The drawing under review shows one solid part. Ordinate dimensions are in mm from its lowest x, y, z. Coordinates: 2 decimals unless noted, no trailing zeros. Order: outer loops, then holes, each group sorted by start corner. A loop starts at its lowest first (then second) coordinate and runs counter-clockwise, first axis right, second up. Notation, with made-up numbers: (19.5, 49) - (36.5, 49) arc R25 ccw to (36.5, 82) - close; hole circle Ø11 at (66, 71.25). An arc over 180 degrees is marked (long way). Answer in a Markdown table with one row per item.
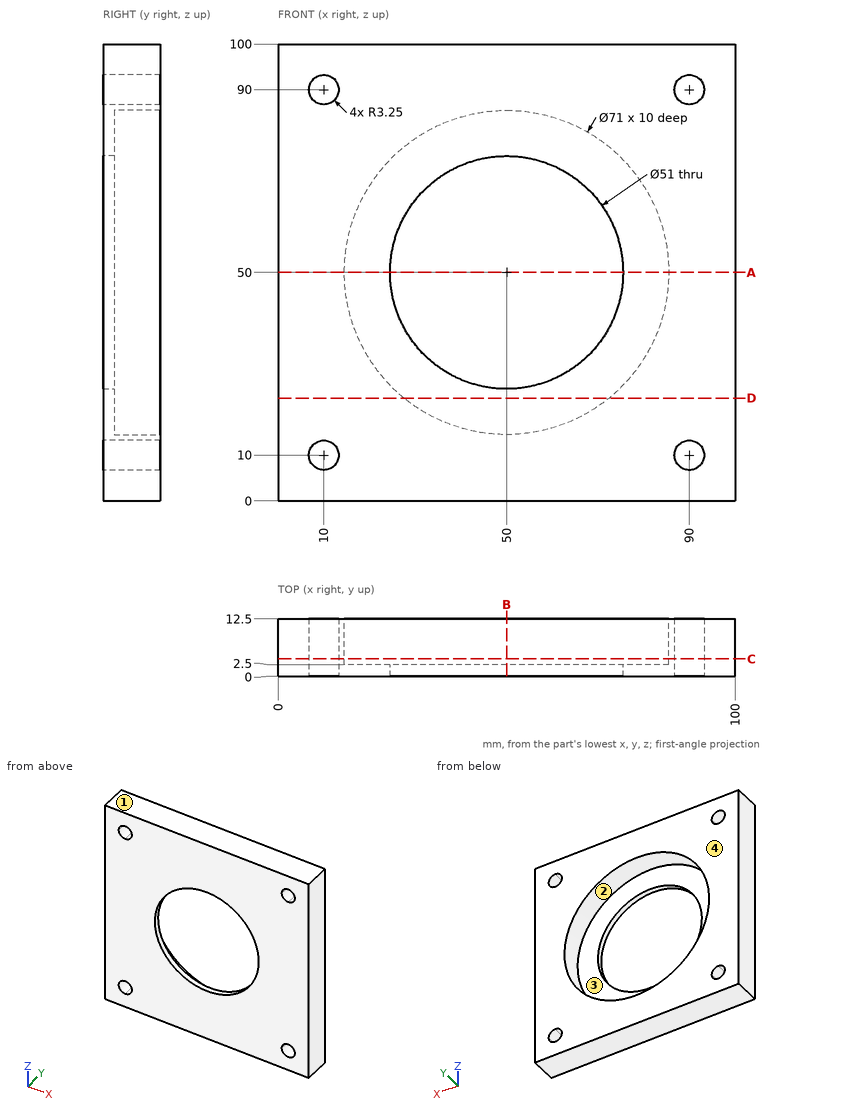
Item 1: Clearance check with a flat-ended pin moving along its axis: pin 1 Ø21.5 at (x, z) = (54, 58) entering from +Y. State where the tip first meets the part, or that it passes through.
Check values:
| item | result |
|---|---|
| pin 1 | through |
Item 2: We need section D-D, the plane z = 22.5. Write out the cut boundary in (x, y), then the cut area to 3 significant figures.
Check values:
| item | result |
|---|---|
| outline | (0, 0) - (100, 0) - (100, 12.5) - (72.45, 12.5) - (72.45, 2.5) - (27.55, 2.5) - (27.55, 12.5) - (0, 12.5) - close |
| area | 801 mm^2 |
Item 3: To check wall thickness, follow line 1 (X direction, y = 0.9, z = 50); line 2 (X direction, y = 5.5, z = 50); line 3 (Z direction, x = 12, y = 0.5). State the ranges of each line that lie inside material, in increasing order. Write a range as from..to.
Check values:
| item | result |
|---|---|
| line 1 | 0..24.5, 75.5..100 |
| line 2 | 0..14.5, 85.5..100 |
| line 3 | 0..7.44, 12.56..87.44, 92.56..100 |
Item 4: We need section C-C, the plane y = 3.75. Write out the cut boundary in (x, z).
Check values:
| item | result |
|---|---|
| outline | (0, 0) - (100, 0) - (100, 100) - (0, 100) - close; hole circle Ø6.5 at (10, 10); hole circle Ø6.5 at (10, 90); hole circle Ø71 at (50, 50); hole circle Ø6.5 at (90, 10); hole circle Ø6.5 at (90, 90) |
Item 5: Mouldability with a two-part tool opening along Z and no side actions: class the marked faces 1, 2, 3 and 4 as +Z half, -Z half, draft (parallel to the pull), parting line (faces both ways), or undercut.
Check values:
| item | result |
|---|---|
| face 1 | +Z half |
| face 2 | undercut |
| face 3 | undercut |
| face 4 | draft |
Item 6: We need section A-A, the plane z = 50. Write out the cut boundary in (x, y).
Check values:
| item | result |
|---|---|
| outline | (0, 0) - (24.5, 0) - (24.5, 2.5) - (14.5, 2.5) - (14.5, 12.5) - (0, 12.5) - close; (75.5, 0) - (100, 0) - (100, 12.5) - (85.5, 12.5) - (85.5, 2.5) - (75.5, 2.5) - close |
Item 7: We need section B-B, the plane x = 50. Write out the cut boundary in (y, z).
Check values:
| item | result |
|---|---|
| outline | (0, 0) - (12.5, 0) - (12.5, 14.5) - (2.5, 14.5) - (2.5, 24.5) - (0, 24.5) - close; (0, 75.5) - (2.5, 75.5) - (2.5, 85.5) - (12.5, 85.5) - (12.5, 100) - (0, 100) - close |
